```python
from build123d import *

# Parameters (mm, degrees)
F0_W     = 914.4
F0_H     = 838.2
F1_DEPTH = 1778
F2_W     = 914.4
F2_H     = 609.6
F2_W_2   = 445.77
F2_H_2   = 1140.46
F2_W_3   = 457.2
F3_DEPTH = 76.2
F4_R     = 12.7


with BuildPart() as f1:
    # F0 (on Top) → F1 (new body)
    with BuildSketch(Plane.XY):
        with Locations((-457.2, -419.1)):
            Rectangle(F0_W, F0_H)
    extrude(amount=F1_DEPTH)

    # F2 (on face) → F3 (join)
    with BuildSketch(Plane.XZ.offset(838.2)):
        with Locations((-457.2, 304.8)):
            Rectangle(F2_W, F2_H)
        with Locations((-688.975, 1205.23)):
            Rectangle(F2_W_2, F2_H_2)
        with Locations((-231.14, 1205.23)):
            Rectangle(F2_W_3, F2_H_2)
    extrude(amount=F3_DEPTH)

    # F4
    f4_edges = [f1.edges().sort_by_distance(p)[0] for p in [
        (-688.975, -914.4, 1775.46),
        (-466.09, -914.4, 1205.23),
        (-459.74, -914.4, 1205.23),
        (-231.14, -914.4, 1775.46),
        (-2.54, -914.4, 1205.23),
        (-231.14, -914.4, 635),
        (-688.975, -914.4, 635),
        (-911.86, -914.4, 1205.23),
        (-457.2, -914.4, 609.6),
        (-914.4, -914.4, 304.8),
        (-457.2, -914.4, 0),
        (0, -914.4, 304.8),
    ]]
    fillet(f4_edges, radius=F4_R)


solid = f1.part
```
Geometry: final body of the model. Coordinates: model frame, mm. A direction names the side the tool comes from. Round coordinates to 2 decimals unless told otherwise and drop trailing zeros. Answer in a Markdown table with one row per item. Add a question column.
(1) Draft query along Z for faces 6 (the face through (-692, -870, 635)), 7 (the face through (-464, -445, 0)), 8 (the face through (-911.86, -870, 1197)), 9 (the face through (-692, -870, 1775.46)). Return one class per face: pulls with the +Z half, pulls with the -Z half, needs draft (parallel to the pull), parting line crosses it, or undercut.
(2) Reachability of faces 1 (the face through (-2.54, -870, 1197)), 2 (the face through (-464, -870, 609.6)), 3 (the face through (-234, -870, 1775.46)), 4 (the face through (-459.74, -870, 1197)), 5 (the face through (-692, -914.4, 1213)) from +Z, -Z, +X, -X, +Y, -Y: full face, straight path, thin tool, end or side. Return the list, or none.
(3) Ray query, L1, parallel to Z at x = -176.5, y = -847.5. Return the intervals inside material, ascending.
Established:
| question | item | result |
|---|---|---|
| 1 | face 6 | undercut |
| 1 | face 7 | pulls with the -Z half |
| 1 | face 8 | needs draft |
| 1 | face 9 | pulls with the +Z half |
| 2 | face 1 | +Z, +X, -Y |
| 2 | face 2 | +X, -X, -Y |
| 2 | face 3 | +Z, +X, -X, -Y |
| 2 | face 4 | +Z, -Y |
| 2 | face 5 | +Z, -Z, +X, -X, -Y |
| 3 | L1 | 0 to 609.6, 635 to 1775.46 |
